Can you work these out from the model? Positions are in its coordinate system, mm. Face numbers are marked on the shaded views. Round coordinates to 2 decimals unless told otherwise and drop trailing zeros. Loops run counter-clockwise (first coordinate to the right, second up) from the corner with the lowest first, then second, coordinate; pieces in that order, holes last.
(1) If I drill on line 1 along Z through (x, y) = (0, -11); line 2 along Y through (x, z) = (7, 0), over which ranges is the centre line in solid material (lowest first)?
(2) I want a section at A-A on z = 0. Write out the boundary of the cut face in (x, y), plus the area to 3 significant figures.
(3) Thinking about a two-plate mould opening in Z: for the marked faces 1 and 2, which applies, released by +Z, released by -Z, zero draft, split by the parting line, or undercut?
(4) Will these pins go through, and if not, where does the flat tip stop? pin 1 Ø4 at (x, z) = (14.5, 0.5) entering from +Y; pin 2 Ø2 at (y, z) = (-63, 4) entering from -X; pin 3 Ø8 at (y, z) = (-53.5, -14.5) entering from -X.
(5) I want a section at B-B on y = 15. Write out the boundary of the cut face in (x, z).
(6) I want a section at C-C on x = -56. Write out the boundary of the cut face in (y, z), plus the area to 3 significant figures.
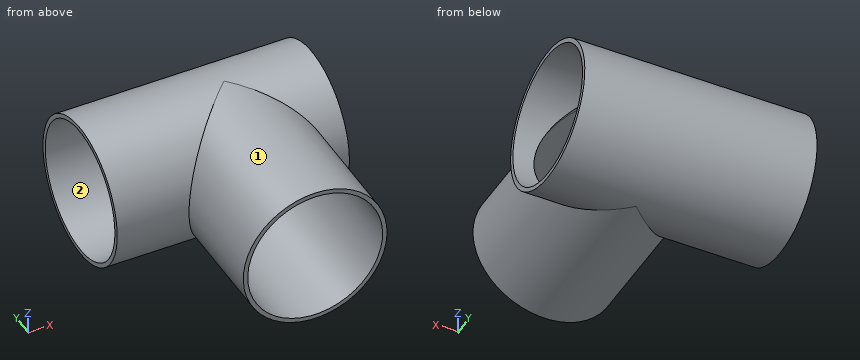
from build123d import *
from build123d.topology import SkipClean

# Parameters (mm, degrees)
BOSS_EXTRUDE1_DEPTH      = 40
BOSS_EXTRUDE1_DEPTH_BACK = 40
SKETCH1_R                = 32.5
SKETCH1_R_2              = 30.5
SKETCH2_R                = 32.5
SKETCH2_R_2              = 30.5
BOSS_EXTRUDE2_DEPTH      = 80
SKETCH3_R                = 30.5
CUT_EXTRUDE1_DEPTH       = 80
CUT_EXTRUDE2_START       = -79
SKETCH4_R                = 30.5
CUT_EXTRUDE2_DEPTH       = 79
SKETCH5_R                = 32.5
SKETCH5_R_2              = 30.5
BOSS_EXTRUDE3_DEPTH      = 25


with BuildPart() as part:
    # Sketch1 → Boss-Extrude1 (new, two sides: drawn at the far end of the back side and taken through both)
    with BuildSketch(Plane(origin=(0, 0, 0), x_dir=(0, 0, -1), z_dir=(1, 0, 0)).offset(-BOSS_EXTRUDE1_DEPTH_BACK)):
        Circle(SKETCH1_R)
        Circle(SKETCH1_R_2, mode=Mode.SUBTRACT)
    extrude(amount=BOSS_EXTRUDE1_DEPTH + BOSS_EXTRUDE1_DEPTH_BACK)

    # Sketch2 → Boss-Extrude2 (add)
    with BuildSketch(Plane(origin=(0, 0, 0), x_dir=(1, 0, 0), z_dir=(0, 1, 0))):
        with Locations(Location((0, 0, 0), (0, 0, 270))):
            Circle(SKETCH2_R)
        with Locations(Location((0, 0, 0), (0, 0, 270))):
            Circle(SKETCH2_R_2, mode=Mode.SUBTRACT)
    extrude(amount=-BOSS_EXTRUDE2_DEPTH)

    # Sketch3 → Cut-Extrude1 (cut)
    with SkipClean():  # the faces are left unmerged after this step: merging them gives an invalid solid
        with BuildSketch(Plane(origin=(40, 0, 0), x_dir=(0, 0, -1), z_dir=(1, 0, 0))):
            Circle(SKETCH3_R)
        extrude(amount=-CUT_EXTRUDE1_DEPTH, mode=Mode.SUBTRACT)

    # Sketch4 → Cut-Extrude2 (cut)
    with SkipClean():  # the faces are left unmerged after this step: merging them gives an invalid solid
        with BuildSketch(Plane.XZ.offset(80).offset(CUT_EXTRUDE2_START)):
            with Locations(Location((0, 0, 0), (0, 0, 90))):
                Circle(SKETCH4_R)
        extrude(amount=CUT_EXTRUDE2_DEPTH, mode=Mode.SUBTRACT)

    # Sketch5 → Boss-Extrude3 (add)
    with SkipClean():  # the faces are left unmerged after this step: merging them gives an invalid solid
        with BuildSketch(Plane.ZY.offset(40)):
            with Locations(Location((0, 0, 0), (0, 0, 180))):
                Circle(SKETCH5_R)
            with Locations(Location((0, 0, 0), (0, 0, 180))):
                Circle(SKETCH5_R_2, mode=Mode.SUBTRACT)
        extrude(amount=BOSS_EXTRUDE3_DEPTH)


solid = part.part
Filled sheet:
1. line 1: z = -32.5 to -30.5, 30.5 to 32.5
1. line 2: y = 30.5 to 32.5
2. outline: (-65, -32.5) - (-32.5, -32.5) - (-32.5, -80) - (-30.5, -80) - (-30.5, -30.5) - (-65, -30.5) - close; (-65, 30.5) - (40, 30.5) - (40, 32.5) - (-65, 32.5) - close; (30.5, -80) - (32.5, -80) - (32.5, -32.5) - (40, -32.5) - (40, -30.5) - (30.5, -30.5) - close
2. area: 488 mm2
3. face 1: split by the parting line
3. face 2: undercut
4. pin 1: stops at y = 32.5
4. pin 2: stops at x = -32.36
4. pin 3: stops at x = -30.76
5. outline: (-65, -28.83) - (40, -28.83) - (40, -26.56) - (-65, -26.56) - close; (-65, 26.56) - (40, 26.56) - (40, 28.83) - (-65, 28.83) - close
6. outline: circle Ø65 at (0, 0); hole circle Ø61 at (0, 0)
6. area: 396 mm2
